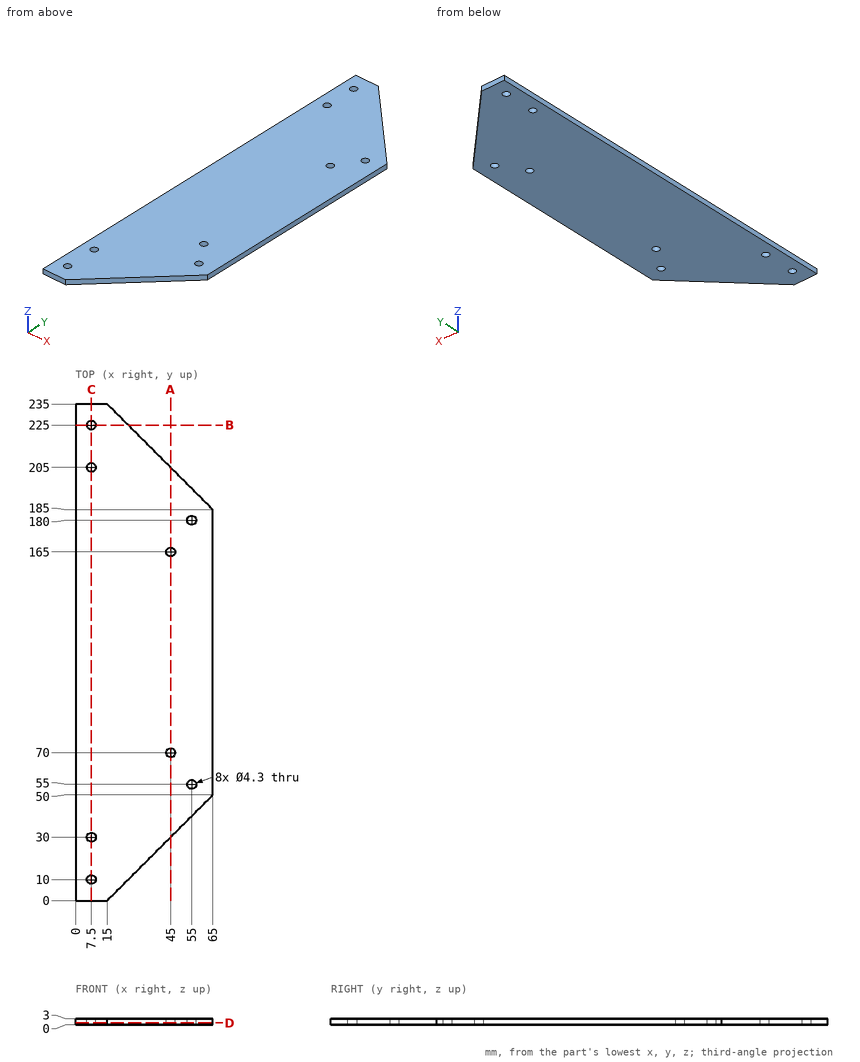
The figure shows three views and two pictorial views of one solid part (mm, origin at its lowest corner). Answer the questions. Coordinates: 2 decimals unless noted, no trailing zeros. Loops run counter-clockwise (first coordinate to the right, second up) from the corner with the lowest first, then second, coordinate; pieces in that order, holes last.
1) Find section A-A on x = 45. Write down the section's boundary in (y, z).
2) Find section C-C on x = 7.5. Write down the section's boundary in (y, z).
3) Find section D-D on z = 1. Give the number of separate pieces and of enclosed holes in the cut face, then the cut area to 3 significant figures.
4) Find the intervals of material crossed by L1, parallel to Y at x = 45, z = 0.85; L2, parallel to X at y = 180, z = 2.05; L3, parallel to Y at x = 55, z = 0.8, in increasing order.
5) Find section B-B on y = 225. Write down the section's boundary in (x, z).
Values:
1. outline: (30, 0) - (67.85, 0) - (67.85, 3) - (30, 3) - close; (72.15, 0) - (162.85, 0) - (162.85, 3) - (72.15, 3) - close; (167.15, 0) - (205, 0) - (205, 3) - (167.15, 3) - close
2. outline: (0, 0) - (7.85, 0) - (7.85, 3) - (0, 3) - close; (12.15, 0) - (27.85, 0) - (27.85, 3) - (12.15, 3) - close; (32.15, 0) - (202.85, 0) - (202.85, 3) - (32.15, 3) - close; (207.15, 0) - (222.85, 0) - (222.85, 3) - (207.15, 3) - close; (227.15, 0) - (235, 0) - (235, 3) - (227.15, 3) - close
3. separate pieces: 1
3. enclosed holes: 8
3. area: 12,700 mm2
4. L1: y = 30 to 67.85, 72.15 to 162.85, 167.15 to 205
4. L2: x = 0 to 52.85, 57.15 to 65
4. L3: y = 40 to 52.85, 57.15 to 177.85, 182.15 to 195
5. outline: (0, 0) - (5.35, 0) - (5.35, 3) - (0, 3) - close; (9.65, 0) - (25, 0) - (25, 3) - (9.65, 3) - close
